Part print with two shaded views. Sizes in mm from the minimum x, y, z corner. A direction names the side the tool comes from. Give positions to 0.01 mm unless a question says otherwise; leave off trailing zeros. Loops run counter-clockwise (first coordinate to the right, second up) from the corner with the lowest first, then second, coordinate; pieces in that order, holes last. Notation, with made-up numbers: M -22.75,23.5 L 23.25,23.5 A16 cw 23.25,53.5 Z; hole C 33.25,-37.75 d7. An arc over 180 degrees is marked long. Answer as a JSON object with one key per item and string values. Group by question number.
1. 3-axis set-ups, long thin cutter, end or side, ignore diameter. For the marked faces 1 and 2: which of +Z, -Z, +X, -X, +Y, -Y reach the whole face in a straight line?
2. Slice it at A-A (y = 170). List the corners of the cut face in (x, z).
3. Slice it at D-D (y = 30). List the corners of the cut face in (x, z), then the cut area to 3 significant figures.
4. Slice it at C-C (x = 81). List the corners of the cut face in (y, z).
5. Slice it at B-B (z = 9). List the corners of the cut face in (x, y), then the cut area to 3 significant figures.
6. Drill centre lines: line 1 along Z through (x, y) = (118.5, 30); line 2 along Z through (x, y) = (55, 170); line 3 along X through (y, z) = (91, 80.5). Where is each one in solid material? Low to high. Write a range as [from, to].
7. Drop flat-ended pins along their axis: pin 1 Ø16.5 at (x, z) = (12, 72) entering from -Y; pin 2 Ø4 at (x, z) = (55, 68) entering from -Y. Give the stop position or say it passes through.
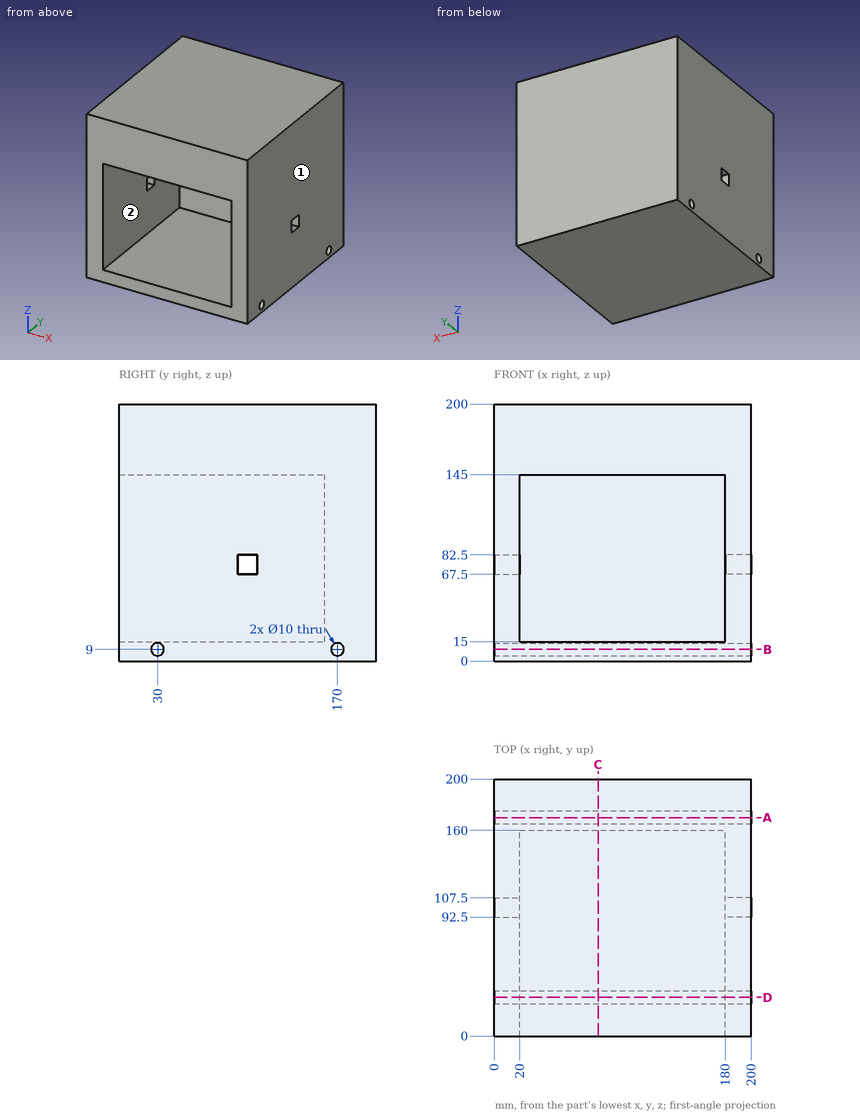
Established:
{
 "1": {"face 1": "+Z, -Z, +X, +Y, -Y", "face 2": "-Y"},
 "2": {"outline": "M 0,0 L 200,0 L 200,4 L 0,4 Z; M 0,14 L 200,14 L 200,200 L 0,200 Z"},
 "3": {"outline": "M 0,0 L 200,0 L 200,4 L 0,4 Z; M 0,14 L 200,14 L 200,200 L 0,200 Z; hole M 20,15 L 180,15 L 180,145 L 20,145 Z", "area": "17,200 mm^2"},
 "4": {"outline": "M 0,0 L 200,0 L 200,200 L 0,200 L 0,145 L 160,145 L 160,15 L 0,15 Z; hole C 30,9 d10; hole C 170,9 d10"},
 "5": {"outline": "M 0,0 L 200,0 L 200,25 L 0,25 Z; M 0,35 L 200,35 L 200,165 L 0,165 Z; M 0,175 L 200,175 L 200,200 L 0,200 Z", "area": "36,000 mm^2"},
 "6": {"line 1": "z = [0, 4], [14, 15], [145, 200]", "line 2": "z = [0, 4], [14, 200]", "line 3": "x = [0, 20], [180, 200]"},
 "7": {"pin 1": "stops at y = 0", "pin 2": "stops at y = 160"}
}
